Read the model definition and answer for the solid it produces. Units are mm, in the model's axes. Coordinates: 2 decimals unless noted, no trailing zeros. Order: outer loops, then holes, each group sorted by start corner. A loop starts at its lowest first (then second) coordinate and runs counter-clockwise, first axis right, second up. Notation, with made-up numbers: M -21,20.5 L 29,20.5 A32 ccw 29,47.5 Z; hole C 29,6.5 d6. An arc over 180 degrees is marked long. Put each result on its own line as item: value.
from build123d import *

# Parameters (mm, degrees)
SKETCH1_R           = 4
BOSS_EXTRUDE1_DEPTH = 147
FILLET1_R           = 0.5
SKETCH2_W           = 6.178297582
SKETCH2_H           = 2
CUT_EXTRUDE1_DEPTH  = 20


with BuildPart() as part:
    # Sketch1 → Boss-Extrude1 (new body)
    with BuildSketch(Plane(origin=(0, 0, 0), x_dir=(0, 0, -1), z_dir=(1, 0, 0))):
        Circle(SKETCH1_R)
    extrude(amount=BOSS_EXTRUDE1_DEPTH)

    # Fillet1
    fillet1_edges = [part.edges().sort_by_distance(p)[0] for p in [
        (0, 0, 4),
        (147, 0, 4),
    ]]
    fillet(fillet1_edges, radius=FILLET1_R)

    # Sketch2 → Cut-Extrude1 (cut)
    with BuildSketch(Plane.ZY):
        with Locations((0, 4)):
            Rectangle(SKETCH2_W, SKETCH2_H)
    extrude(amount=-CUT_EXTRUDE1_DEPTH, mode=Mode.SUBTRACT)


solid = part.part
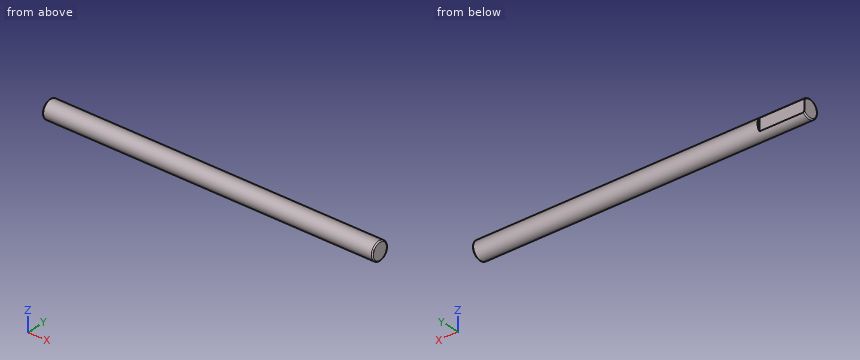
Q1. Consider line 1 along Y through (x, z) = (76, -3); line 2 along X through (y, z) = (-2.75, -2.5). Determine where each line is inside the solid, lowest interval first.
Answers below:
line 1: y = -2.65 to 2.65
line 2: x = 0.05 to 146.95
Q2. Find section B-B on x = 31.5. Write down the section's boundary in (y, z), plus the area to 3 significant figures.
Answers below:
outline: C 0,0 d8
area: 50.3 mm^2
Q3. Find section A-A on z = 0. Write down the section's boundary in (x, y).
Answers below:
outline: M 0,-3.5 A0.5 ccw 0.5,-4 L 146.5,-4 A0.5 ccw 147,-3.5 L 147,3.5 A0.5 ccw 146.5,4 L 20,4 L 20,3 L 0,3 Z
Q4. Given pin 1 (1 mm diameter, centred on x = 76.5, z = 1.5, fed in from +Y); pin 2 (1 mm diameter, centred on x = 117, y = 2.5, fed in from +Z); pin 3 (2.5 mm diameter, centred on x = 11.5, z = -1.5, fed in from +Y), each flat-ended and moving along its own axis, determine where each tip first touches the part or whether it passes through.
Answers below:
pin 1: stops at y = 3.87
pin 2: stops at z = 3.46
pin 3: stops at y = 3
